The drawing under review shows one solid part. Ordinate dimensions are in mm from its lowest x, y, z. Give positions to 0.01 mm unless a question says otherwise; leave off trailing zeros. Loops run counter-clockwise (first coordinate to the right, second up) from the corner with the lowest first, then second, coordinate; pieces in that order, holes last. Notation, with made-up numbers: (-38, -26) -> (10, -26) arc R26 cw to (10, 8) -> close; hole circle Ø8 at (47.25, -21). An arc over 180 degrees is marked (long way). Answer in a Markdown table with one row per item. Add a question column.
(1) For pin 1 (1.5 mm diameter, centred on x = 6, z = 5, fed in from -Y); pin 2 (1 mm diameter, centred on x = 11.5, z = 5, fed in from -Y) (3 decimals); pin 3 (2 mm diameter, centred on x = 2, z = 5, fed in from +Y); pin 4 (4 mm diameter, centred on x = 8.5, y = 9, fed in from -Z), all flat-tipped, find the tip position at first contact; note any pin that passes through.
(2) Consider section C-C on z = 2.5. Write out the cut boundary in (x, y), then the cut area to 3 significant figures.
(3) Consider section A-A on x = 9. Write out the cut boundary in (y, z).
(4) Draft analysis for pull direction X (two halves, no side actions). For the marked faces 1, 2 and 3, state which applies: +X half, -X half, draft (parallel to the pull), parting line (faces both ways), or undercut.
(5) For line 1 (Y direction, x = 9, z = 5.5); line 2 (X direction, y = 9.75, z = 0.75); line 3 (X direction, y = 6, z = 5) (1 decimal), list the stretches that pass through material, from the lowest coordinate up.
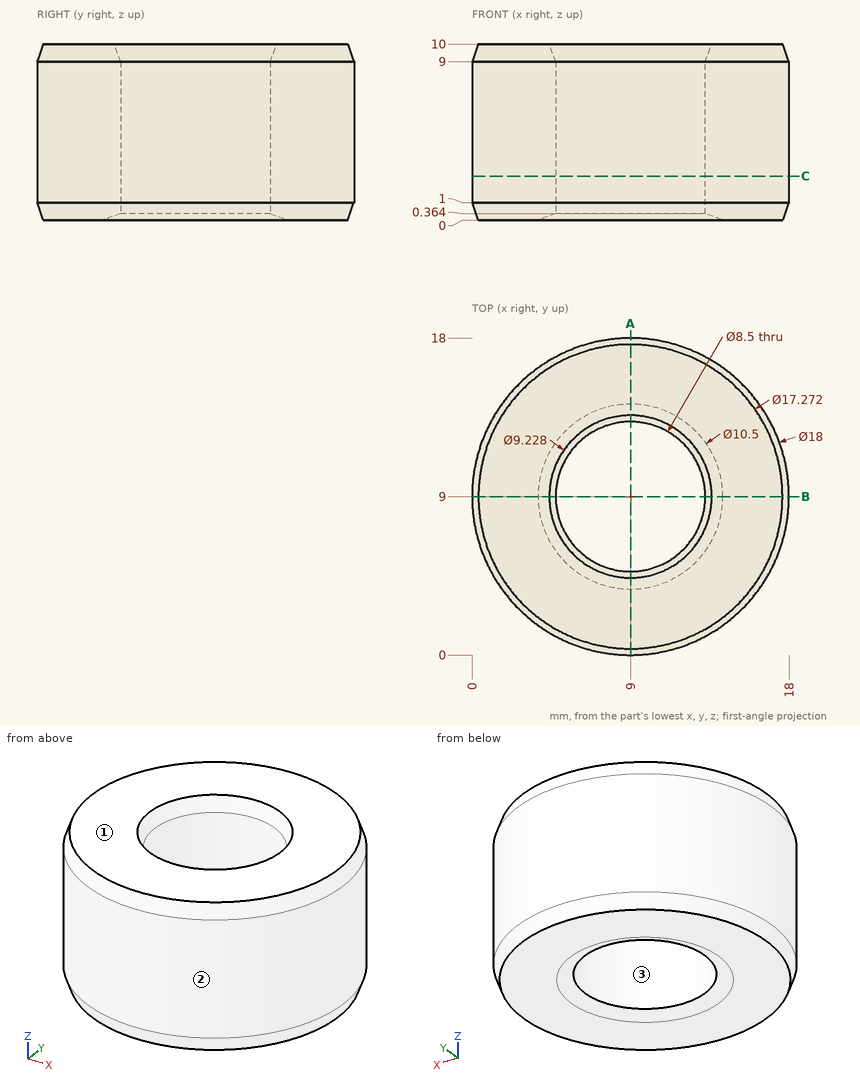
Values follow:
| question | item | result |
|---|---|---|
| 1 | pin 1 | y = 0.29 |
| 1 | pin 2 | y = 0.225 |
| 1 | pin 3 | y = 15.71 |
| 1 | pin 4 | through |
| 2 | outline | circle Ø18 at (9, 9); hole circle Ø8.5 at (9, 9) |
| 2 | area | 198 mm2 |
| 3 | outline | (0, 1) -> (0.36, 0) -> (3.75, 0) -> (4.75, 0.36) -> (4.75, 9) -> (4.39, 10) -> (0.36, 10) -> (0, 9) -> close; (13.25, 0.36) -> (14.25, 0) -> (17.64, 0) -> (18, 1) -> (18, 9) -> (17.64, 10) -> (13.61, 10) -> (13.25, 9) -> close |
| 4 | face 1 | draft |
| 4 | face 2 | parting line |
| 4 | face 3 | undercut |
| 5 | line 1 | 0 to 4.75, 13.25 to 18 |
| 5 | line 2 | 0.12 to 4.82, 13.18 to 17.88 |
| 5 | line 3 | 0.5 to 6, 12 to 17.5 |
